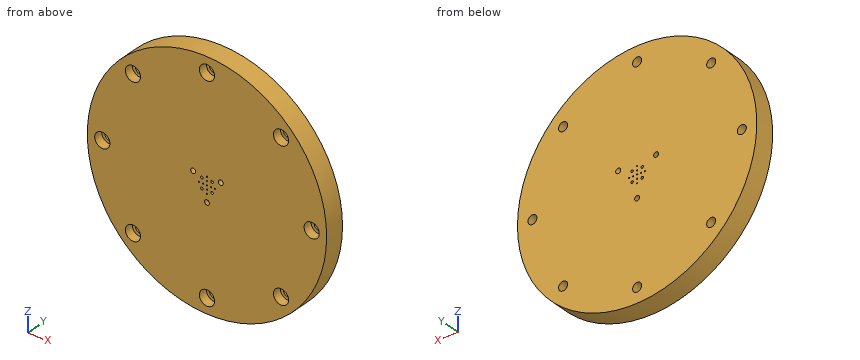
```python
from build123d import *

# Parameters (mm, degrees)
SKETCH1_R                                      = 38.1
BOSS_EXTRUDE1_DEPTH                            = 6.35
CBORE_FOR_4_BUTTON_HEAD_CAP_SCREW1_D           = 2.8702
CBORE_FOR_4_BUTTON_HEAD_CAP_SCREW1_CBORE_D     = 4.826
CBORE_FOR_4_BUTTON_HEAD_CAP_SCREW1_CBORE_DEPTH = 2.794
CIRPATTERN1_COUNT                              = 8
SKETCH6_R                                      = 0.1984375
CUT_EXTRUDE1_DEPTH                             = 7.35
CIRPATTERN2_COUNT                              = 4
SKETCH6_3_R                                    = 0.1984375
CUT_EXTRUDE2_DEPTH                             = 7.35
SKETCH6_5_R                                    = 0.408305
CUT_EXTRUDE4_DEPTH                             = 7.35
CIRPATTERN4_COUNT                              = 4
SKETCH7_R                                      = 0.79375
CIRPATTERN6_COUNT                              = 3


with BuildPart() as part:
    # Sketch1 → Boss-Extrude1 (new body)
    with BuildSketch(Plane(origin=(0, 0, 0), x_dir=(1, 0, 0), z_dir=(0, 1, 0))):
        Circle(SKETCH1_R)
    extrude(amount=BOSS_EXTRUDE1_DEPTH)

    # CBORE for _4 Button Head Cap Screw1 (through all)
    with Locations(Plane(origin=(0, 0, 0), x_dir=(-1, 0, 0), z_dir=(0, -1, 0))):
        with Locations((0, -33.3375)):
            cbore_for_4_button_head_cap_screw1 = CounterBoreHole(CBORE_FOR_4_BUTTON_HEAD_CAP_SCREW1_D / 2, CBORE_FOR_4_BUTTON_HEAD_CAP_SCREW1_CBORE_D / 2, CBORE_FOR_4_BUTTON_HEAD_CAP_SCREW1_CBORE_DEPTH)

    # CirPattern1: CBORE for _4 Button Head Cap Screw1 ×8 about axis
    cirpattern1_axis = Axis((0, 0, 0), (0, 1, 0))
    for i in range(1, CIRPATTERN1_COUNT):
        add(cbore_for_4_button_head_cap_screw1.rotate(cirpattern1_axis, i * 360 / CIRPATTERN1_COUNT), mode=Mode.SUBTRACT)

    # Sketch6 → Cut-Extrude1 (cut, through all)
    with BuildSketch(Plane.XZ):
        with Locations((0, -2.54)):
            Circle(SKETCH6_R)
        with Locations((0, -1.27)):
            Circle(SKETCH6_R)
    cut_extrude1 = extrude(amount=-CUT_EXTRUDE1_DEPTH, mode=Mode.SUBTRACT)

    # CirPattern2: Cut-Extrude1 ×4 about axis
    cirpattern2_axis = Axis((0, 0, 0.000106785), (0, 1, 0))
    for i in range(1, CIRPATTERN2_COUNT):
        add(cut_extrude1.rotate(cirpattern2_axis, i * 360 / CIRPATTERN2_COUNT), mode=Mode.SUBTRACT)

    # Sketch6_3 → Cut-Extrude2 (cut, through all)
    with BuildSketch(Plane.XZ):
        Circle(SKETCH6_3_R)
    extrude(amount=-CUT_EXTRUDE2_DEPTH, mode=Mode.SUBTRACT)

    # Sketch6_5 → Cut-Extrude4 (cut, through all)
    with BuildSketch(Plane.XZ):
        with Locations((1.616446102, -1.616446102)):
            Circle(SKETCH6_5_R)
    cut_extrude4 = extrude(amount=-CUT_EXTRUDE4_DEPTH, mode=Mode.SUBTRACT)

    # CirPattern4: Cut-Extrude4 ×4 about axis
    cirpattern4_axis = Axis((0, 0, 0), (0, 1, 0))
    for i in range(1, CIRPATTERN4_COUNT):
        add(cut_extrude4.rotate(cirpattern4_axis, i * 360 / CIRPATTERN4_COUNT), mode=Mode.SUBTRACT)

    # Cut-Sweep1: sweep along a curve in space
    with BuildLine() as cut_sweep1_path:
        Line((0, 6.35, -6.985), (0, 0, -5.08))
    # Sketch7 → Cut-Sweep1 (sweep, cut)
    with BuildSketch(Plane(origin=(0, 6.35, 0), x_dir=(1, 0, 0), z_dir=(0, 1, 0))):
        with Locations((0, 6.985)):
            Circle(SKETCH7_R)
    cut_sweep1 = sweep(path=cut_sweep1_path.line, mode=Mode.SUBTRACT)

    # CirPattern6: Cut-Sweep1 ×3 about axis
    cirpattern6_axis = Axis((0, 6.35, 0), (0, -1, 0))
    for i in range(1, CIRPATTERN6_COUNT):
        add(cut_sweep1.rotate(cirpattern6_axis, i * 360 / CIRPATTERN6_COUNT), mode=Mode.SUBTRACT)


solid = part.part
```
Verification items for the finished model (mm, model axes). Round coordinates to 2 decimals unless told otherwise and drop trailing zeros. Order: outer loops, then holes, each group sorted by start corner. A loop starts at its lowest first (then second) coordinate and runs counter-clockwise, first axis right, second up.
1) Cross-section at A-A, the plane y = 5.25. Give the number of separate pieces and of enclosed holes in the cut face, plus the area to 3 significant figures.
Geometry says:
separate pieces: 1
enclosed holes: 24
area: 4,500 mm2
2) Material ranges on line 1 (Z direction, x = -1.5, y = 5.25); line 2 (Z direction, x = -25.5, y = 2.75); line 3 (X direction, y = 5, z = 3.5), recorded low to high.
Geometry says:
line 1: z = -38.07 to -2.01, -1.23 to 1.23, 2.01 to 38.07
line 2: z = -28.31 to -25.03, -22.12 to 22.12, 25.03 to 28.31
line 3: x = -37.94 to -6.46, -4.93 to 4.93, 6.46 to 37.94
3) Cross-section at B-B, the plane x = 10. Record the cut outline in (y, z).
Geometry says:
outline: (0, -36.76) - (6.35, -36.76) - (6.35, 36.76) - (0, 36.76) - close
4) Depth check by flat-ended pin: pin 1 (2 mm diameter, centred on y = 1, z = -9, fed in from +X); pin 2 (2 mm diameter, centred on x = -13.5, y = 5.5, fed in from -Z); pin 3 (2.5 mm diameter, centred on x = 0, z = 33, fed in from -Y); pin 4 (2.5 mm diameter, centred on x = -33.34, z = 0, fed in from -Y). Enter the tip coordinate at first touch or a pass-through.
Geometry says:
pin 1: stops at x = 37.25
pin 2: stops at z = -35.99
pin 3: stops at y = 2.79
pin 4: passes through
5) Cross-section at C-C, the plane z = 20. Record the cut outline in (x, y).
Geometry says:
outline: (-32.43, 0) - (32.43, 0) - (32.43, 6.35) - (-32.43, 6.35) - close
